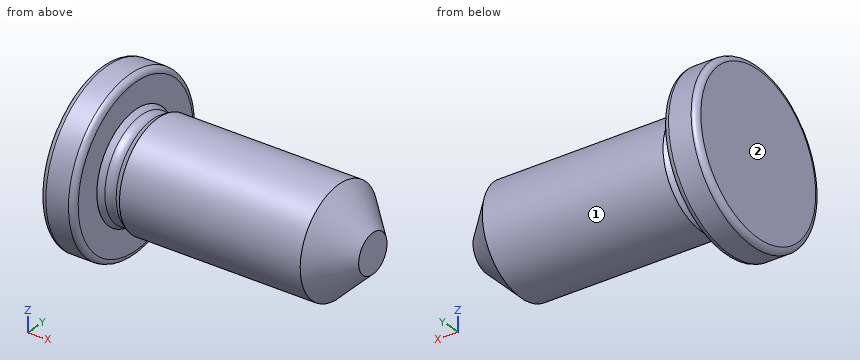
from build123d import *

# Parameters (mm, degrees)
F0_W     = 19
F0_H     = 4.72735
F2_R     = 1
F3_R     = 0.5
F4_SIZE2 = 3
F4_SIZE  = 3


with BuildPart() as f1:
    # F0 (on Front) → F1 (revolve)
    with BuildSketch(Plane.XZ):
        Polygon((0, 7.5), (0, 0), (3, 0), (3, 4.72735), (3, 7.5), align=None)
        Polygon((3, 4.72735), (3, 0), (4, 0), (4, 4.15), align=None)
        Polygon((4, 4.15), (4, 0), (5, 0), (5, 4.72735), align=None)
        with Locations((14.5, 2.363675)):
            Rectangle(F0_W, F0_H)
    revolve(axis=Axis((12, 0, 0), (1, 0, 0)))

    # F2
    f2_edges = [f1.edges().sort_by_distance(p)[0] for p in [
        (4, 0, -4.15),
    ]]
    fillet(f2_edges, radius=F2_R)

    # F3
    f3_edges = [f1.edges().sort_by_distance(p)[0] for p in [
        (0, 0, -7.5),
        (3, 0, -7.5),
    ]]
    fillet(f3_edges, radius=F3_R)

    # F4
    f4_edges = [f1.edges().sort_by_distance(p)[0] for p in [
        (24, 0, -4.72735),
    ]]
    chamfer(f4_edges, length=F4_SIZE, length2=F4_SIZE2)


solid = f1.part
Can you work these out from the model? Positions are in its coordinate system, mm. Face numbers are marked on the shaded views. A direction names the side the tool comes from. Round coordinates to 2 decimals unless told otherwise and drop trailing zeros. Write each loop counter-clockwise with the first axis right and the second up, starting at its lowest first coordinate (ties: lowest second). Pieces come first, ordered by that corner, then holes. Notation, with made-up numbers: (65, -7) -> (94, -7) arc R20 cw to (94, -2) -> close; hole circle Ø1 at (-38, -40). An arc over 180 degrees is marked (long way). One line per question, with ' | ' between items. Start each with the question number.
1) I'm going to push flat-ended pins straight in: P1, Ø4, axis at x = 6, z = -4.5, coming from the -Y side; P2, Ø1, axis at y = -6, z = -5, coming from the +X side; P3, Ø4, axis at y = -5, z = 0.5, coming from the +X side. Where does each tip first touch, or does it pass through?
2) Suppose I cut it at A-A on x = 9.75. Write out the boundary of the cut face in (y, z), then the cut area to 3 significant figures.
3) On a 3-axis mill with a long thin cutter (end or side, diameter ignored), from which of +Z, -Z, +X, -X, +Y, -Y can I reach the whole of each face in a straight line? I mean the marked faces 1 and 2. Say none if no direction works.
4) I need wall thicknesses on line 1 (X direction, y = -2.25, z = 6); line 2 (Z direction, x = 12.5, y = 0); line 3 (X direction, y = 2.25, z = -2.5). Which ranges of each line are inside material? Lowest first, please. Write a range as [from, to].
5) Suppose I cut it at B-B on x = 21.5. Write out the boundary of the cut face in (y, z).
Return value:
1) P1: stops at y = -4.01 | P2: stops at x = 2.89 | P3: stops at x = 22.7
2) outline: circle Ø9.45 at (0, 0) | area: 70.2 mm2
3) face 1: +X | face 2: +Z, -Z, -X, +Y, -Y
4) line 1: x = [0, 3] | line 2: z = [-4.73, 4.73] | line 3: x = [0, 22.36]
5) outline: circle Ø8.45 at (0, 0)
